```python
from build123d import *

# Parameters (mm, degrees)
SKETCH1_W           = 77.4
SKETCH1_H           = 67
SKETCH1_W_2         = 65.4
SKETCH1_H_2         = 55
BOSS_EXTRUDE1_DEPTH = 14
SKETCH2_R           = 2.75
CUT_EXTRUDE1_DEPTH  = 6
SKETCH3_R           = 2.75
CUT_EXTRUDE2_DEPTH  = 6


with BuildPart() as part:
    # Sketch1 → Boss-Extrude1 (new body)
    with BuildSketch(Plane(origin=(0, 0, 0), x_dir=(1, 0, 0), z_dir=(0, 1, 0))):
        Rectangle(SKETCH1_W, SKETCH1_H)
        Rectangle(SKETCH1_W_2, SKETCH1_H_2, mode=Mode.SUBTRACT)
    extrude(amount=BOSS_EXTRUDE1_DEPTH)

    # Sketch2 → Cut-Extrude1 (cut)
    with BuildSketch(Plane(origin=(38.7, 0, 0), x_dir=(0, 0, -1), z_dir=(1, 0, 0))):
        with Locations((-20.75, 7)):
            Circle(SKETCH2_R)
        with Locations((20.75, 7)):
            Circle(SKETCH2_R)
    extrude(amount=-CUT_EXTRUDE1_DEPTH, mode=Mode.SUBTRACT)

    # Sketch3 → Cut-Extrude2 (cut)
    with BuildSketch(Plane(origin=(-32.7, 0, 0), x_dir=(0, 0, -1), z_dir=(1, 0, 0))):
        with Locations((15.85, 7)):
            Circle(SKETCH3_R)
        with Locations((-15.85, 7)):
            Circle(SKETCH3_R)
    extrude(amount=-CUT_EXTRUDE2_DEPTH, mode=Mode.SUBTRACT)


solid = part.part
```
Here's how the part is built. I have some questions about the finished solid (model axes, mm). A direction names the side the tool comes from. Round coordinates to 2 decimals unless told otherwise and drop trailing zeros. Order: outer loops, then holes, each group sorted by start corner. A loop starts at its lowest first (then second) coordinate and runs counter-clockwise, first axis right, second up. Notation, with made-up numbers: (54.25, 20) -> (83.25, 20) arc R10 ccw to (83.25, 38) -> close; hole circle Ø6 at (85, -34). An arc over 180 degrees is marked (long way). Use a Markdown table: item, result. Add a question column.
(1) Suppose I cut it at A-A, the plane z = -11.5. Please give me the cut outline in (x, y), and give its area (3 significant figures).
(2) Suppose I cut it at C-C, the plane z = 15.85. Please give me the cut outline in (x, y).
(3) Suppose I cut it at B-B, the plane y = 7. Please give me the cut outline in (x, z), and give its area (3 significant figures).
(4) For faces 5 (the face through (32.7, 7, 0)), 6 (the face through (-35.66, 5.95, -18.39)), 7 (the face through (-1, 0, 29)), 8 (the face through (35.7, 7.1, 23.5)), which set-ups out of +Z, -Z, +X, -X, +Y, -Y let a thin tool reach every point of the face, with its end or its side?
(5) I need wall thicknesses on line 1 along Z through (x, y) = (-29.5, 7.5); line 2 along X through (y, z) = (2.5, 6); line 3 along Y through (x, z) = (-37.25, -15.85). Which ranges of each line are inside material? Lowest first, please.
(6) Suppose I cut it at D-D, the plane x = -21. Please give me the cut outline in (y, z).
(7) For pin 1 Ø8 at (x, z) = (25, -12.5) entering from +Y, with a flat end and sliding along its axis, tell me the tip position at first contact or that it passes through.
(8) If we mould it in two halves opening along X, with no side actions, what happens to faces 1 (the face through (-32.7, 7, 0)), 2 (the face through (38.7, 7, 0)), 3 (the face through (-35.66, 4.56, 14.58)), 4 (the face through (-38.7, 7, 0))? For each: released by +X, released by -X, zero draft, split by the parting line, or undercut.
Verdict:
| question | item | result |
|---|---|---|
| 1 | outline | (-38.7, 0) -> (-32.7, 0) -> (-32.7, 14) -> (-38.7, 14) -> close; (32.7, 0) -> (38.7, 0) -> (38.7, 14) -> (32.7, 14) -> close |
| 1 | area | 168 mm2 |
| 2 | outline | (-38.7, 0) -> (-32.7, 0) -> (-32.7, 4.25) -> (-38.7, 4.25) -> close; (-38.7, 9.75) -> (-32.7, 9.75) -> (-32.7, 14) -> (-38.7, 14) -> close; (32.7, 0) -> (38.7, 0) -> (38.7, 14) -> (32.7, 14) -> close |
| 3 | outline | (-38.7, -33.5) -> (38.7, -33.5) -> (38.7, -23.5) -> (32.7, -23.5) -> (32.7, -27.5) -> (-32.7, -27.5) -> (-32.7, -18.6) -> (-38.7, -18.6) -> close; (-38.7, -13.1) -> (-32.7, -13.1) -> (-32.7, 13.1) -> (-38.7, 13.1) -> close; (-38.7, 18.6) -> (-32.7, 18.6) -> (-32.7, 27.5) -> (32.7, 27.5) -> (32.7, 23.5) -> (38.7, 23.5) -> (38.7, 33.5) -> (-38.7, 33.5) -> close; (32.7, -18) -> (38.7, -18) -> (38.7, 18) -> (32.7, 18) -> close |
| 3 | area | 1,460 mm2 |
| 4 | face 5 | +Y, -Y |
| 4 | face 6 | -X |
| 4 | face 7 | +Z, -Z, +X, -X, -Y |
| 4 | face 8 | +X |
| 5 | line 1 | -33.5 to -27.5, 27.5 to 33.5 |
| 5 | line 2 | -38.7 to -32.7, 32.7 to 38.7 |
| 5 | line 3 | 0 to 4.25, 9.75 to 14 |
| 6 | outline | (0, -33.5) -> (14, -33.5) -> (14, -27.5) -> (0, -27.5) -> close; (0, 27.5) -> (14, 27.5) -> (14, 33.5) -> (0, 33.5) -> close |
| 7 | pin 1 | through |
| 8 | face 1 | undercut |
| 8 | face 2 | released by +X |
| 8 | face 3 | zero draft |
| 8 | face 4 | released by -X |
